from build123d import *

# Parameters (mm, degrees)
SKETCH_1_W           = 35
SKETCH_1_H           = 20
EXTRUDE_1_DEPTH      = 8
SKETCH_2_W           = 29
SKETCH_2_H           = 14
CUT_EXTRUDE_2_DEPTH  = 0.8
SKETCH_3_W           = 29
SKETCH_3_H           = 7.2
CUT_EXTRUDE_4_DEPTH  = 42.097445176
SKETCH_4_W           = 6
SKETCH_4_H           = 6
CUT_EXTRUDE_5_DEPTH  = 42.097445176
SKETCH_5_R           = 1.3
CUT_EXTRUDE_6_DEPTH  = 42.097445176
CUT_EXTRUDE_START    = 8
CUT_EXTRUDE_8_DEPTH  = 50.097445176
SKETCH_6_R           = 2.2
CUT_EXTRUDE_10_DEPTH = 2
SKETCH_8_W           = 35
SKETCH_8_H           = 20
CUT_EXTRUDE_11_DEPTH = 3


with BuildPart() as part:
    # 草圖1 → 填料-伸長1 (new body)
    with BuildSketch(Plane(origin=(0, 0, 0), x_dir=(1, 0, 0), z_dir=(0, 1, 0))):
        with Locations((17.5, 10)):
            Rectangle(SKETCH_1_W, SKETCH_1_H)
    extrude(amount=EXTRUDE_1_DEPTH)

    # 草圖2 → 除料-伸長2 (cut)
    with BuildSketch(Plane(origin=(0, 0, 0), x_dir=(1, 0, 0), z_dir=(0, 1, 0))):
        with Locations((20.5, 7)):
            Rectangle(SKETCH_2_W, SKETCH_2_H)
    extrude(amount=CUT_EXTRUDE_2_DEPTH, mode=Mode.SUBTRACT)

    # 草圖3 → 除料-伸長4 (cut, through all)
    with BuildSketch(Plane(origin=(0, 0, 0), x_dir=(1, 0, 0), z_dir=(0, 1, 0))):
        with Locations((20.5, 3.6)):
            Rectangle(SKETCH_3_W, SKETCH_3_H)
    extrude(amount=CUT_EXTRUDE_4_DEPTH, mode=Mode.SUBTRACT)

    # 草圖4 → 除料-伸長5 (cut, through all)
    with BuildSketch(Plane(origin=(0, 0, 0), x_dir=(1, 0, 0), z_dir=(0, 1, 0))):
        with Locations((32, 17)):
            Rectangle(SKETCH_4_W, SKETCH_4_H)
    extrude(amount=CUT_EXTRUDE_5_DEPTH, mode=Mode.SUBTRACT)

    # 草圖5 → 除料-伸長6 (cut, through all)
    with BuildSketch(Plane(origin=(0, 0, 0), x_dir=(1, 0, 0), z_dir=(0, 1, 0))):
        with Locations(Location((3, 16, 0), (0, 0, 270))):
            Circle(SKETCH_5_R)
        with Locations(Location((3, 4, 0), (0, 0, 270))):
            Circle(SKETCH_5_R)
        with Locations(Location((9, 16, 0), (0, 0, 270))):
            Circle(SKETCH_5_R)
        with Locations(Location((26, 16, 0), (0, 0, 270))):
            Circle(SKETCH_5_R)
    extrude(amount=CUT_EXTRUDE_6_DEPTH, mode=Mode.SUBTRACT)

    # 草圖7 → 除料-伸長8 (cut, through all)
    with BuildSketch(Plane(origin=(0, 0, 0), x_dir=(1, 0, 0), z_dir=(0, 1, 0)).offset(CUT_EXTRUDE_START)):
        Polygon((26, 18.4), (23.921539031, 17.2), (23.921539031, 14.8), (26, 13.6), (28.078460969, 14.8), (28.078460969, 17.2), align=None)
        Polygon((9, 18.4), (6.921539031, 17.2), (6.921539031, 14.8), (9, 13.6), (11.078460969, 14.8), (11.078460969, 17.2), align=None)
    extrude(amount=-CUT_EXTRUDE_8_DEPTH, mode=Mode.SUBTRACT)

    # 草圖6 → 除料-伸長10 (cut)
    with BuildSketch(Plane(origin=(0, 0, 0), x_dir=(1, 0, 0), z_dir=(0, 1, 0))):
        with Locations(Location((3, 16, 0), (0, 0, 90))):
            Circle(SKETCH_6_R)
        with Locations(Location((3, 4, 0), (0, 0, 90))):
            Circle(SKETCH_6_R)
    extrude(amount=CUT_EXTRUDE_10_DEPTH, mode=Mode.SUBTRACT)

    # 草圖8 → 除料-伸長11 (cut)
    with BuildSketch(Plane(origin=(0, 0, 0), x_dir=(1, 0, 0), z_dir=(0, 1, 0))):
        with Locations((17.5, 10)):
            Rectangle(SKETCH_8_W, SKETCH_8_H)
    extrude(amount=CUT_EXTRUDE_11_DEPTH, mode=Mode.SUBTRACT)


solid = part.part
Work out the finished part from the listing and answer in its coordinate system (mm). A direction names the side the tool comes from. Give positions to 0.01 mm unless a question says otherwise; leave off trailing zeros. Loops run counter-clockwise (first coordinate to the right, second up) from the corner with the lowest first, then second, coordinate; pieces in that order, holes last. Notation, with made-up numbers: (17.25, 32.25) - (25.25, 32.25) arc R18 ccw to (25.25, 44.25) - close; hole circle Ø7 at (77.5, 86.5). An arc over 180 degrees is marked (long way). Answer in a Markdown table with one row per item. Add a question column.
Q1. The part is cut by section D-D (y = 4.25). Determine the outline of the cut face in (x, z).
Q2. A tool of negligible diameter and unlimited length cuts with its end or side. For faces 4 (the flat face through (29, 5, -17)), 5 (the flat face through (35, 5, -11)), 6 (the flat face through (7.946, 5.535, -14.208)), from which of +Z, -Z, +X, -X, +Y, -Y can it reach the whole face along a straight path? Write none if from no direction.
Q3. The part is cut by section C-C (z = -4). Determine the outline of the cut face in (x, y), and give its area (3 significant figures).
Q4. Determine the mould class of faces 1 (the flat face through (23.922, 6, -16)), 2 (the flat face through (14, 5, -20)), 3 (the flat face through (20, 5, -7.2)) for opening direction Z: released by +Z, released by -Z, zero draft, split by the parting line, or undercut.
Q5. The part is cut by section B-B (z = -16). Determine the outline of the cut face in (x, y).
Q6. Each of these flat-tipped pins is pushed along its axis until it touches: P1, Ø1.5, axis at x = 13.5, y = 5, coming from the +Z side; P2, Ø1.5, axis at y = 6, z = -15.5, coming from the +X side; P3, Ø1, axis at x = 28, z = -5, coming from the -Y side. Where does it stop, or does it pass through?
Q7. Consider line 1 along Z through (x, y) = (3, 6.3); line 2 along X through (y, z) = (4.55, -16); line 3 along X through (y, z) = (5.85, -15.5). Determine where each line is inside the solid, lowest interval first.
Q8. The part is cut by section A-A (x = 3). Determine the outline of the cut face in (y, z).
Solution:
| question | item | result |
|---|---|---|
| 1 | outline | (0, -20) - (29, -20) - (29, -14) - (35, -14) - (35, -7.2) - (6, -7.2) - (6, 0) - (0, 0) - close; hole circle Ø2.6 at (3, -16); hole circle Ø2.6 at (3, -4); hole (6.92, -17.2) - (9, -18.4) - (11.08, -17.2) - (11.08, -14.8) - (9, -13.6) - (6.92, -14.8) - close; hole (23.92, -17.2) - (26, -18.4) - (28.08, -17.2) - (28.08, -14.8) - (26, -13.6) - (23.92, -14.8) - close |
| 2 | face 4 | -Z, +X, +Y, -Y |
| 2 | face 5 | +Z, -Z, +X, +Y, -Y |
| 2 | face 6 | +Y, -Y |
| 3 | outline | (0, 3) - (1.7, 3) - (1.7, 8) - (0, 8) - close; (4.3, 3) - (6, 3) - (6, 8) - (4.3, 8) - close |
| 3 | area | 17.0 mm² |
| 4 | face 1 | undercut |
| 4 | face 2 | released by -Z |
| 4 | face 3 | released by +Z |
| 5 | outline | (0, 3) - (1.7, 3) - (1.7, 8) - (0, 8) - close; (4.3, 3) - (6.92, 3) - (6.92, 8) - (4.3, 8) - close; (11.08, 3) - (23.92, 3) - (23.92, 8) - (11.08, 8) - close; (28.08, 3) - (29, 3) - (29, 8) - (28.08, 8) - close |
| 6 | P1 | stops at z = -7.2 |
| 6 | P2 | stops at x = 29 |
| 6 | P3 | passes through |
| 7 | line 1 | z = -20 to -17.3, -14.7 to -5.3, -2.7 to 0 |
| 7 | line 2 | x = 0 to 1.7, 4.3 to 6.92, 11.08 to 23.92, 28.08 to 29 |
| 7 | line 3 | x = 0 to 1.8, 4.2 to 6.92, 11.08 to 23.92, 28.08 to 29 |
| 8 | outline | (3, -20) - (8, -20) - (8, -17.3) - (3, -17.3) - close; (3, -14.7) - (8, -14.7) - (8, -5.3) - (3, -5.3) - close; (3, -2.7) - (8, -2.7) - (8, 0) - (3, 0) - close |
